Could you check a few things on this drawing? It's one solid part, dimensions in mm from its lowest x, y, z. A direction names the side the tool comes from. Coordinates: 2 decimals unless noted, no trailing zeros. Write each loop counter-clockwise with the first axis right and the second up, starting at its lowest first coordinate (ties: lowest second). Pieces come first, ordered by that corner, then holes.
Item 1: I want a section at A-A (z = 7.25). Please give me the cut outline in (x, y).
Item 2: I want a section at B-B (z = 2.75). Please give me the cut outline in (x, y).
Item 3: I want a section at C-C (x = 23.9). Please give me the cut outline in (y, z).
Item 4: I'm going to push flat-ended pins straight in: P1, Ø0.7, axis at x = 28, y = 12, coming from the -Z side; P2, Ø4.5, axis at x = 23.9, y = 7.9, coming from the +Z side. Where does each tip first touch, or does it pass through?
Item 5: For the marked faces 4, 5 and 6, which set-ups out of +Z, -Z, +X, -X, +Y, -Y let a thin tool reach every point of the face, with its end or its side?
Item 6: Please list where these lines run through material, in increasing order: line 1 (Y direction, x = 7.9, z = 4); line 2 (X direction, y = 3.9, z = 9.1) (3 decimals); line 3 (X direction, y = 2.75, z = 5.25).
Item 7: If we mould it in two halves opening along Y, with no side actions, what happens to the marked faces 1, 2 and 3? For each: pulls with the +Y half, pulls with the -Y half, needs draft (parallel to the pull), parting line crosses it, or undercut.
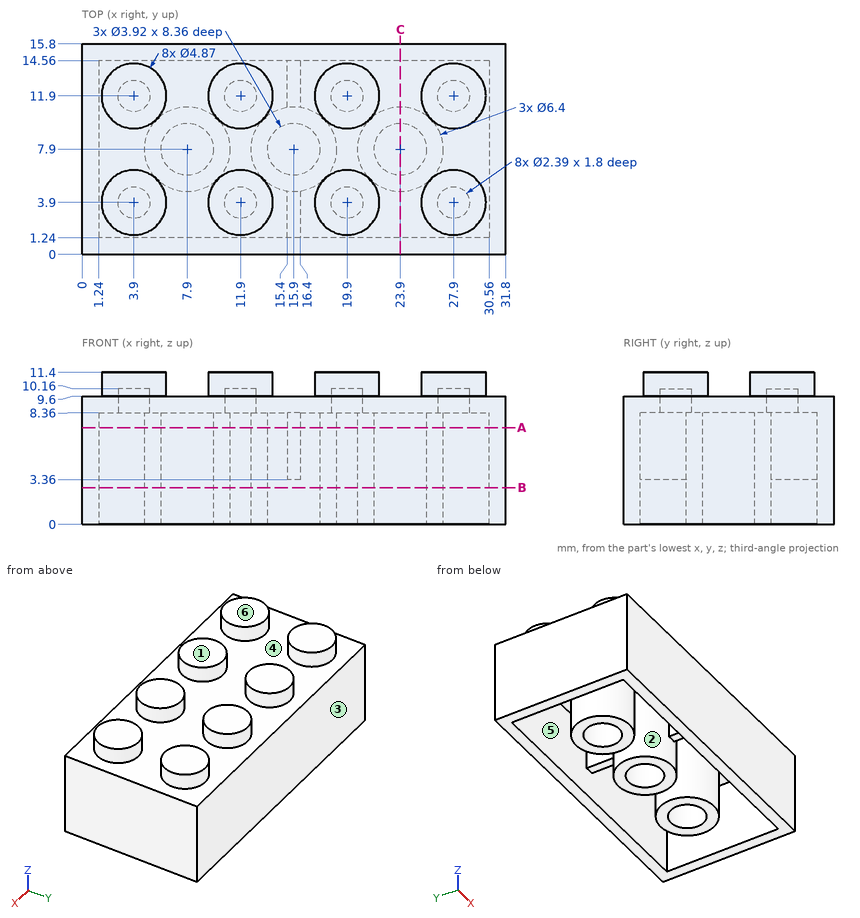
Answer:
1. outline: (0, 0) - (31.8, 0) - (31.8, 15.8) - (0, 15.8) - close; circle Ø6.4 at (7.9, 7.9); circle Ø6.4 at (23.9, 7.9); hole (1.24, 1.24) - (15.4, 1.24) - (15.4, 4.74) arc R3.2 cw to (15.4, 11.06) - (15.4, 14.56) - (1.24, 14.56) - close; hole circle Ø3.92 at (7.9, 7.9); hole circle Ø3.92 at (15.9, 7.9); hole (16.4, 1.24) - (30.56, 1.24) - (30.56, 14.56) - (16.4, 14.56) - (16.4, 11.06) arc R3.2 cw to (16.4, 4.74) - close; hole circle Ø3.92 at (23.9, 7.9)
2. outline: (0, 0) - (31.8, 0) - (31.8, 15.8) - (0, 15.8) - close; circle Ø6.4 at (7.9, 7.9); circle Ø6.4 at (15.9, 7.9); circle Ø6.4 at (23.9, 7.9); hole (1.24, 1.24) - (30.56, 1.24) - (30.56, 14.56) - (1.24, 14.56) - close; hole circle Ø3.92 at (7.9, 7.9); hole circle Ø3.92 at (15.9, 7.9); hole circle Ø3.92 at (23.9, 7.9)
3. outline: (0, 0) - (1.24, 0) - (1.24, 8.36) - (4.7, 8.36) - (4.7, 0) - (5.94, 0) - (5.94, 8.36) - (9.86, 8.36) - (9.86, 0) - (11.1, 0) - (11.1, 8.36) - (14.56, 8.36) - (14.56, 0) - (15.8, 0) - (15.8, 9.6) - (0, 9.6) - close
4. P1: stops at z = 10.16
4. P2: stops at z = 9.6
5. face 4: +Z
5. face 5: -Z
5. face 6: +Z, +X, -X, +Y, -Y
6. line 1: y = 0 to 1.24, 4.7 to 5.94, 9.86 to 11.1, 14.56 to 15.8
6. line 2: x = 0 to 2.705, 5.095 to 10.705, 13.095 to 18.705, 21.095 to 26.705, 29.095 to 31.8
6. line 3: x = 0 to 1.24, 15.4 to 16.4, 30.56 to 31.8
7. face 1: needs draft
7. face 2: undercut
7. face 3: pulls with the +Y half
